Source: CAD feature listing. Evaluate the final solid. Frame: model axes, mm. A direction names the side the tool comes from. Give positions to 0.01 mm unless a question says otherwise; leave off trailing zeros. Order: outer loops, then holes, each group sorted by start corner. A loop starts at its lowest first (then second) coordinate and runs counter-clockwise, first axis right, second up. Notation, with made-up numbers: (65.25, 38.25) -> (119.25, 38.25) arc R34 cw to (119.25, 70.25) -> close; hole circle Ø9 at (41.5, 13). An arc over 180 degrees is marked (long way). Answer in a Markdown table with one row per item.
```python
from build123d import *

# Parameters (mm, degrees)
F0_R     = 9.525
F1_DEPTH = 9.525
F3_R     = 19.05
F4_DEPTH = 57.15
F7_DEPTH = 57.15


with BuildPart() as f1:
    # F0 (on Front) → F1 (new body, symmetric)
    with BuildSketch(Plane.XZ):
        with BuildLine():
            Line((19.05, 0), (349.25, 0))
            Line((349.25, 0), (349.25, 101.6))
            ThreePointArc((349.25, 101.6), (341.810512, 119.560512), (323.85, 127))
            Line((323.85, 127), (0, 127))
            Line((0, 127), (0, 19.05))
            ThreePointArc((0, 19.05), (13.470384, 13.470384), (19.05, 0))
        make_face()
        with Locations((323.85, 101.6)):
            Circle(F0_R, mode=Mode.SUBTRACT)
        with BuildLine():
            Line((-349.25, 0), (-19.05, 0))
            ThreePointArc((-19.05, 0), (-13.470384, 13.470384), (0, 19.05))
            Line((0, 19.05), (0, 127))
            Line((0, 127), (-323.85, 127))
            ThreePointArc((-323.85, 127), (-341.810512, 119.560512), (-349.25, 101.6))
            Line((-349.25, 101.6), (-349.25, 0))
        make_face()
        with Locations((-323.85, 101.6)):
            Circle(F0_R, mode=Mode.SUBTRACT)
        with BuildLine():
            Line((-323.85, -127), (0, -127))
            Line((0, -127), (0, -19.05))
            ThreePointArc((0, -19.05), (-13.470384, -13.470384), (-19.05, 0))
            Line((-19.05, 0), (-349.25, 0))
            Line((-349.25, 0), (-349.25, -101.6))
            ThreePointArc((-349.25, -101.6), (-341.810512, -119.560512), (-323.85, -127))
        make_face()
        with Locations((-323.85, -101.6)):
            Circle(F0_R, mode=Mode.SUBTRACT)
        with BuildLine():
            Line((0, -127), (323.85, -127))
            ThreePointArc((323.85, -127), (341.810512, -119.560512), (349.25, -101.6))
            Line((349.25, -101.6), (349.25, 0))
            Line((349.25, 0), (19.05, 0))
            ThreePointArc((19.05, 0), (13.470384, -13.470384), (0, -19.05))
            Line((0, -19.05), (0, -127))
        make_face()
        with Locations((323.85, -101.6)):
            Circle(F0_R, mode=Mode.SUBTRACT)
    extrude(amount=F1_DEPTH, both=True)

    # F3 (on offset) → F4 (join)
    with BuildSketch(Plane.YZ.offset(349.25)):
        with BuildLine():
            Line((-47.625, -38.1), (-9.525, -38.1))
            Line((-9.525, -38.1), (-9.525, 0))
            ThreePointArc((-9.525, 0), (-20.684232, -26.940768), (-47.625, -38.1))
        make_face()
        with BuildLine():
            ThreePointArc((-47.625, 38.1), (-20.684232, 26.940768), (-9.525, 0))
            Line((-9.525, 0), (-9.525, 38.1))
            Line((-9.525, 38.1), (-47.625, 38.1))
        make_face()
        with Locations((-47.625, 0)):
            Circle(F3_R)
        with BuildLine():
            ThreePointArc((-47.625, -38.1), (-20.684232, -26.940768), (-9.525, 0))
            ThreePointArc((-9.525, 0), (-20.684232, 26.940768), (-47.625, 38.1))
            ThreePointArc((-47.625, 38.1), (-85.725, 0), (-47.625, -38.1))
        make_face()
        with Locations((-47.625, 0)):
            Circle(F3_R, mode=Mode.SUBTRACT)
    extrude(amount=-F4_DEPTH)

    # F6 (on offset) → F7 (join)
    with BuildSketch(Plane(origin=(-349.25, 0, 0), x_dir=(0, -1, 0), z_dir=(-1, 0, 0))):
        with BuildLine():
            ThreePointArc((47.625, 38.1), (20.684232, 26.940768), (9.525, 0))
            ThreePointArc((9.525, 0), (20.684232, -26.940768), (47.625, -38.1))
            ThreePointArc((47.625, -38.1), (74.565768, -26.940768), (85.725, 0))
            ThreePointArc((85.725, 0), (74.565768, 26.940768), (47.625, 38.1))
        make_face()
        with BuildLine():
            ThreePointArc((66.675, 0), (47.625, -19.05), (28.575, 0))
            ThreePointArc((28.575, 0), (47.625, 19.05), (66.675, 0))
        make_face(mode=Mode.SUBTRACT)
        with BuildLine():
            Line((9.525, 38.1), (9.525, 0))
            ThreePointArc((9.525, 0), (20.684232, 26.940768), (47.625, 38.1))
            Line((47.625, 38.1), (9.525, 38.1))
        make_face()
        with BuildLine():
            Line((9.525, 0), (9.525, -38.1))
            Line((9.525, -38.1), (47.625, -38.1))
            ThreePointArc((47.625, -38.1), (20.684232, -26.940768), (9.525, 0))
        make_face()
    extrude(amount=-F7_DEPTH)


solid = f1.part
```
(1) Ray query, probe 1 along Z at (x, y) = (323, -3); probe 2 along X at (y, z) = (-5, -98); probe 3 along Y at (x, z) = (212, 66) (3 decimals). Return the intervals inside material, ascending.
A:
| item | result |
|---|---|
| probe 1 | z = -127 to -111.09, -92.11 to 92.11, 111.09 to 127 |
| probe 2 | x = -349.25 to -332.67, -315.03 to 315.03, 332.67 to 349.25 |
| probe 3 | y = -9.525 to 9.525 |
(2) Section query B-B (y = -39). Return the cut outline in (x, z).
A:
| item | result |
|---|---|
| outline | (-349.25, -38.1) -> (-292.1, -38.1) -> (-292.1, -16.99) -> (-349.25, -16.99) -> close; (-349.25, 16.99) -> (-292.1, 16.99) -> (-292.1, 38.1) -> (-349.25, 38.1) -> close; (292.1, -38.1) -> (349.25, -38.1) -> (349.25, -16.99) -> (292.1, -16.99) -> close; (292.1, 16.99) -> (349.25, 16.99) -> (349.25, 38.1) -> (292.1, 38.1) -> close |
(3) Section query C-C (x = 94.5). Return the cut outline in (y, z) (3 decimals), plus the area to 3 significant figures.
A:
| item | result |
|---|---|
| outline | (-9.525, -127) -> (9.525, -127) -> (9.525, 127) -> (-9.525, 127) -> close |
| area | 4,840 mm^2 |
(4) Pull-direction query (Z, two-part tool) for faces 1 (the flat face through (-5, 9.525, 30)), 2 (the cylindrical face through (321.075, -29.455, 5.722)), 3 (the cylindrical face through (341.61, -0.13, -119.76)); classes: +Z half, -Z half, draft (parallel to the pull), parting line (faces both ways), or undercut.
A:
| item | result |
|---|---|
| face 1 | draft |
| face 2 | undercut |
| face 3 | -Z half |
(5) Section query A-A (x = -303.5). Return the cut outline in (y, z) (3 decimals).
A:
| item | result |
|---|---|
| outline | (-85.725, 0) arc R38.1 ccw to (-47.625, -38.1) -> (-9.525, -38.1) -> (-9.525, -127) -> (9.525, -127) -> (9.525, 127) -> (-9.525, 127) -> (-9.525, 38.1) -> (-47.625, 38.1) arc R38.1 ccw to start; hole circle Ø38.1 at (-47.625, 0) |
(6) Access query for faces 4 (the flat face through (321, -28, 38.1)), 5 (the cylindrical face through (332.65, 0.13, -105.25)), 6 (the flat face through (-292.1, -30, 9)), 7 (the flat face through (-321, -28, -38.1)), 8 (the flat face through (-5, 0, -127)). Directions: +Z, -Z, +X, -X, +Y, -Y. A direction counts if a zero-diameter tool reaches every point of the face in a straight line with its end or side. Return the directions, or none.
A:
| item | result |
|---|---|
| face 4 | +Z, +X, -X, -Y |
| face 5 | +Y, -Y |
| face 6 | +Z, -Z, -Y |
| face 7 | -Z, +X, -X, -Y |
| face 8 | -Z, +X, -X, +Y, -Y |
(7) First-contact query: pin 1 Ø19 at (x, y) = (-325, -32.5) entering from +Z; pin 2 Ø25 at (x, z) = (-323.85, 101.6) entering from -Y (3 decimals); pin 3 Ø22 at (x, z) = (323.85, -101.6) entering from +Y (3 decimals). Flat tips, straight axial feed; report the tip coordinate or a pass-through.
A:
| item | result |
|---|---|
| pin 1 | stops at z = 38.1 |
| pin 2 | stops at y = -9.525 |
| pin 3 | stops at y = 9.525 |
